Verification items for this drawing (mm, ordinates from the low corner). A direction names the side the tool comes from. Round coordinates to 2 decimals unless told otherwise and drop trailing zeros. Order: outer loops, then holes, each group sorted by start corner. A loop starts at its lowest first (then second) coordinate and runs counter-clockwise, first axis right, second up. Notation, with made-up numbers: (9, 79.25) -> (41, 79.25) arc R25 ccw to (41, 113.25) -> close; hole circle Ø1 at (-31.75, 13.25). An arc over 180 degrees is marked (long way). Answer in a Markdown table with one row per item.
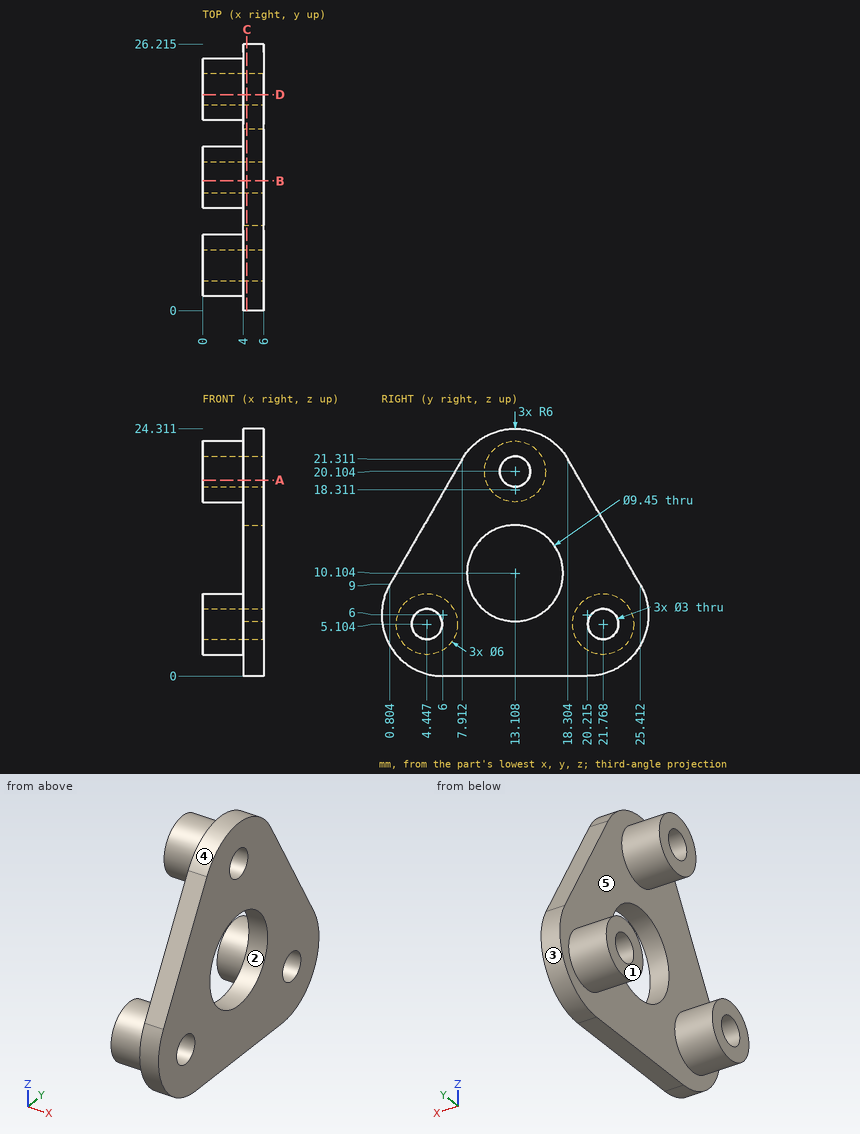
Item 1: Set-up check for the marked faces 4 and 5: record each of +Z, -Z, +X, -X, +Y, -Y from which the full face is reachable in a straight line by a thin tool's end or side.
Result sheet:
| item | result |
|---|---|
| face 4 | +Z, +X, -X |
| face 5 | -X |
Item 2: Scan lines: line 1 (X direction, y = 9.75, z = 22); line 2 (Z direction, x = 2.35, y = 5) (1 decimal); line 3 (Z direction, x = 1.05, y = 4.5) (1 decimal). Record each from-to range of solid material in increasing order. Write a range as [from, to].
Result sheet:
| item | result |
|---|---|
| line 1 | x = [4, 6] |
| line 2 | z = [2.2, 3.7], [6.5, 8.1] |
| line 3 | z = [2.1, 3.6], [6.6, 8.1] |
Item 3: Depth check by flat-ended pin: P1, Ø1.5, axis at y = 8.5, z = 22, coming from the -X side; P2, Ø1.5, axis at x = 3.5, z = 7, coming from the -Y side; P3, Ø3, axis at x = 1.5, z = 4.5, coming from the -Y side. Enter the tip coordinate at first touch or a pass-through.
Result sheet:
| item | result |
|---|---|
| P1 | stops at x = 4 |
| P2 | stops at y = 0.02 |
| P3 | stops at y = 1.45 |
Item 4: Cross-section at D-D (y = 21.25). Record the boundary of the cut face in (x, z) (1 decimal).
Result sheet:
| item | result |
|---|---|
| outline | (0, 2.1) -> (4, 2.1) -> (4, 0.1) -> (6, 0.1) -> (6, 3.7) -> (0, 3.7) -> close; (0, 6.5) -> (6, 6.5) -> (6, 16.2) -> (4, 16.2) -> (4, 8.1) -> (0, 8.1) -> close |
Item 5: Cross-section at A-A (z = 19.25). Record the boundary of the cut face in (x, y) (1 decimal).
Result sheet:
| item | result |
|---|---|
| outline | (0, 10.2) -> (4, 10.2) -> (4, 6.7) -> (6, 6.7) -> (6, 11.9) -> (0, 11.9) -> close; (0, 14.3) -> (6, 14.3) -> (6, 19.5) -> (4, 19.5) -> (4, 16) -> (0, 16) -> close |
Item 6: Cross-section at C-C (x = 4.35). State how many separate pieces and enclosed holes the cut face has, and give its area (3 significant figures).
Result sheet:
| item | result |
|---|---|
| separate pieces | 1 |
| enclosed holes | 4 |
| area | 365 mm^2 |
Item 7: Mould release check, pull along Y, two halves, no side actions. Record for the marked faces 1, 2 and 3: pulls with the +Y half, pulls with the -Y half, needs draft (parallel to the pull), parting line crosses it, or undercut.
Result sheet:
| item | result |
|---|---|
| face 1 | needs draft |
| face 2 | undercut |
| face 3 | pulls with the +Y half |
Item 8: Cross-section at B-B (y = 12.75). Record the boundary of the cut face in (x, z) (1 decimal).
Result sheet:
| item | result |
|---|---|
| outline | (0, 17.1) -> (4, 17.1) -> (4, 14.8) -> (6, 14.8) -> (6, 18.6) -> (0, 18.6) -> close; (0, 21.6) -> (6, 21.6) -> (6, 24.3) -> (4, 24.3) -> (4, 23.1) -> (0, 23.1) -> close; (4, 0) -> (6, 0) -> (6, 5.4) -> (4, 5.4) -> close |
